```python
from build123d import *

# Parameters (mm, degrees)
F3_DEPTH       = 12
F8_R           = 1
F9_DEPTH       = 8
F10_R          = 4.5
F11_DEPTH      = 2
F12_R          = 1
F13_REACH      = 37.3532145158
F12_R_2        = 4.5
F14_DEPTH      = 6
F16_END_RADIUS = 1
F15_R          = 1
F16_REACH      = 37.3532145367
F15_R_2        = 4.5
F17_DEPTH      = 6
F19_END_RADIUS = 1
F18_R          = 1
F19_REACH      = 37.3532145367
F18_R_2        = 4.5
F20_DEPTH      = 6
F22_DEPTH      = 25
F23_R          = 17.5
F23_R_2        = 1.5
F23_R_3        = 6.5
F23_R_4        = 4.5
F24_DEPTH      = 15
F25_DEPTH      = 10


with BuildPart() as f3:
    # F2 (on Top) → F3 (new body)
    with BuildSketch(Plane.XY):
        Polygon((25, -14.4337567297), (0, 28.8675134595), (-25, -14.4337567297), align=None)
    extrude(amount=-F3_DEPTH)

    # F3_face (on face) → F6 section 0
    with BuildSketch(Plane.XY, mode=Mode.PRIVATE) as f6_s0:
        Polygon((-25, -14.4337567297), (25, -14.4337567297), (0, 28.8675134595), align=None)
    loft([f6_s0.sketch, Vertex(0, 0, 10)])

    # F8 (on face) → F9 (cut)
    with BuildSketch(Plane(origin=(0, 0, -12), x_dir=(1, 0, 0), z_dir=(0, 0, -1))):
        Circle(F8_R)
    extrude(amount=-F9_DEPTH, mode=Mode.SUBTRACT)

    # F10 (on face) → F11 (cut)
    with BuildSketch(Plane(origin=(0, 0, -12), x_dir=(1, 0, 0), z_dir=(0, 0, -1))):
        Circle(F10_R)
    extrude(amount=-F11_DEPTH, mode=Mode.SUBTRACT)

    f13_end = f3.faces().sort_by_distance((-1, 0, -7))[0]
    # F12 (on face) → F13 (cut, up to a face of the model that its end follows)
    with BuildSketch(Plane(origin=(0, -4.6812183988, 6.7567567568), x_dir=(1, 0, 0), z_dir=(0, -0.5694947975, 0.8219949365))):
        with Locations((0, -4.3050520255)):
            Circle(F12_R)
    f13_long = extrude(amount=-F13_REACH, mode=Mode.PRIVATE)
    add(split(f13_long, bisect_by=f13_end, keep=Keep.BOTTOM, mode=Mode.PRIVATE), mode=Mode.SUBTRACT)

    # F12 (on face) → F14 (cut)
    with BuildSketch(Plane(origin=(0, -4.6812183988, 6.7567567568), x_dir=(1, 0, 0), z_dir=(0, -0.5694947975, 0.8219949365))):
        with Locations((0, -4.3050520255)):
            Circle(F12_R_2)
        with Locations((0, -4.3050520255)):
            Circle(F12_R, mode=Mode.SUBTRACT)
    extrude(amount=-F14_DEPTH, mode=Mode.SUBTRACT)

    f16_end = (Plane(origin=(0, 0, -7), x_dir=(-1, 0, 0), z_dir=(0, 0, -1)) * Cylinder(F16_END_RADIUS, 214.1194850146, mode=Mode.PRIVATE)).faces().sort_by_distance((-1, 0, -7))[0]
    # F15 (on face) → F16 (cut, up to the whole of a round face its end follows)
    with BuildSketch(Plane(origin=(-4.0540540541, 2.3406091994, 6.7567567568), x_dir=(0.8699176724, 0.1614366008, 0.4660273245), z_dir=(-0.4931969619, 0.2847473987, 0.8219949365))):
        with Locations((-3.5228976388, 2.474401982)):
            Circle(F15_R)
    f16_long = extrude(amount=-F16_REACH, mode=Mode.PRIVATE)
    add(split(f16_long, bisect_by=f16_end, keep=Keep.ALL, mode=Mode.PRIVATE).solids().sort_by_distance((-7.1186849681, 4.1099746826, 4.3050520255))[0], mode=Mode.SUBTRACT)

    # F15 (on face) → F17 (cut)
    with BuildSketch(Plane(origin=(-4.0540540541, 2.3406091994, 6.7567567568), x_dir=(0.8699176724, 0.1614366008, 0.4660273245), z_dir=(-0.4931969619, 0.2847473987, 0.8219949365))):
        with Locations((-3.5228976388, 2.474401982)):
            Circle(F15_R_2)
        with Locations((-3.5228976388, 2.474401982)):
            Circle(F15_R, mode=Mode.SUBTRACT)
    extrude(amount=-F17_DEPTH, mode=Mode.SUBTRACT)

    f19_end = (Plane(origin=(0, 0, -7), x_dir=(-1, 0, 0), z_dir=(0, 0, -1)) * Cylinder(F19_END_RADIUS, 214.1194850146, mode=Mode.PRIVATE)).faces().sort_by_distance((-1, 0, -9.9336675042))[0]
    # F18 (on face) → F19 (cut, up to the whole of a round face its end follows)
    with BuildSketch(Plane(origin=(4.0540540541, 2.3406091994, 6.7567567568), x_dir=(0.8699176724, -0.1614366008, -0.4660273245), z_dir=(0.4931969619, 0.2847473987, 0.8219949365))):
        with Locations((3.5228976388, 2.474401982)):
            Circle(F18_R)
    f19_long = extrude(amount=-F19_REACH, mode=Mode.PRIVATE)
    add(split(f19_long, bisect_by=f19_end, keep=Keep.ALL, mode=Mode.PRIVATE).solids().sort_by_distance((7.1186849681, 4.1099746826, 4.3050520255))[0], mode=Mode.SUBTRACT)

    # F18 (on face) → F20 (cut)
    with BuildSketch(Plane(origin=(4.0540540541, 2.3406091994, 6.7567567568), x_dir=(0.8699176724, -0.1614366008, -0.4660273245), z_dir=(0.4931969619, 0.2847473987, 0.8219949365))):
        with Locations((3.5228976388, 2.474401982)):
            Circle(F18_R_2)
        with Locations((3.5228976388, 2.474401982)):
            Circle(F18_R, mode=Mode.SUBTRACT)
    extrude(amount=-F20_DEPTH, mode=Mode.SUBTRACT)

    # F21 (on face) → F22 (cut)
    with BuildSketch(Plane(origin=(0, 0, -12), x_dir=(1, 0, 0), z_dir=(0, 0, -1))):
        with BuildLine():
            Line((3.2541491538, -23.2311617897), (7.5523574637, -15.7864466154))
            ThreePointArc((7.5523574637, -15.7864466154), (0, -17.5), (-7.5523574637, -15.7864466154))
            Line((-7.5523574637, -15.7864466154), (-3.2541491538, -23.2311617897))
            ThreePointArc((-3.2541491538, -23.2311617897), (0, -23.4579701768), (3.2541491538, -23.2311617897))
        make_face()
        with BuildLine():
            ThreePointArc((-9.8952850725, 14.4337567297), (0, 17.5), (9.8952850725, 14.4337567297))
            Line((9.8952850725, 14.4337567297), (18.4917016925, 14.4337567297))
            ThreePointArc((18.4917016925, 14.4337567297), (0, 23.4579701768), (-18.4917016925, 14.4337567297))
            Line((-18.4917016925, 14.4337567297), (-9.8952850725, 14.4337567297))
        make_face()
        with BuildLine():
            ThreePointArc((-17.4476425363, 1.3526898856), (-15.1554445662, 8.75), (-9.8952850725, 14.4337567297))
            Line((-9.8952850725, 14.4337567297), (-18.4917016925, 14.4337567297))
            ThreePointArc((-18.4917016925, 14.4337567297), (-20.3151980943, 11.7289850884), (-21.7458508462, 8.79740506))
            Line((-21.7458508462, 8.79740506), (-17.4476425363, 1.3526898856))
        make_face()
        with BuildLine():
            ThreePointArc((9.8952850725, 14.4337567297), (15.1554445662, 8.75), (17.4476425363, 1.3526898856))
            Line((17.4476425363, 1.3526898856), (21.7458508462, 8.79740506))
            ThreePointArc((21.7458508462, 8.79740506), (20.3151980943, 11.7289850884), (18.4917016925, 14.4337567297))
            Line((18.4917016925, 14.4337567297), (9.8952850725, 14.4337567297))
        make_face()
        with BuildLine():
            Line((0, -28.8675134595), (3.2541491538, -23.2311617897))
            ThreePointArc((3.2541491538, -23.2311617897), (0, -23.4579701768), (-3.2541491538, -23.2311617897))
            Line((-3.2541491538, -23.2311617897), (0, -28.8675134595))
        make_face()
        with BuildLine():
            ThreePointArc((-21.7458508462, 8.79740506), (-20.3151980943, 11.7289850884), (-18.4917016925, 14.4337567297))
            Line((-18.4917016925, 14.4337567297), (-25, 14.4337567297))
            Line((-25, 14.4337567297), (-21.7458508462, 8.79740506))
        make_face()
        with BuildLine():
            ThreePointArc((18.4917016925, 14.4337567297), (20.3151980943, 11.7289850884), (21.7458508462, 8.79740506))
            Line((21.7458508462, 8.79740506), (25, 14.4337567297))
            Line((25, 14.4337567297), (18.4917016925, 14.4337567297))
        make_face()
    extrude(amount=-F22_DEPTH, mode=Mode.SUBTRACT)

    # F23 (on face) → F24 (join)
    with BuildSketch(Plane(origin=(0, 0, -12), x_dir=(1, 0, 0), z_dir=(0, 0, -1))):
        Circle(F23_R)
        with Locations((-10.8253175473, -6.25)):
            Circle(F23_R_2, mode=Mode.SUBTRACT)
        Circle(F23_R_3, mode=Mode.SUBTRACT)
        with Locations((10.8253175473, 6.25)):
            Circle(F23_R_2, mode=Mode.SUBTRACT)
        Circle(F23_R_3)
        Circle(F23_R_4, mode=Mode.SUBTRACT)
    extrude(amount=F24_DEPTH)

    # F25 (add): a face of the model
    f25_faces = [f3.faces().sort_by_distance(p)[0] for p in [
        (-4.3727207794, 0, -10),
    ]]
    extrude(f25_faces, amount=F25_DEPTH)


solid = f3.part
```
Check sheet for the modelled part. Datum: model origin and axes. Units: mm. A direction names the side the tool comes from. Round coordinates to 2 decimals unless told otherwise and drop trailing zeros. Loops run counter-clockwise (first coordinate to the right, second up) from the corner with the lowest first, then second, coordinate; pieces in that order, holes last. Notation, with made-up numbers: (17.5, 46.5) - (60.5, 46.5) arc R25 cw to (60.5, 79.5) - close; hole circle Ø8 at (-26, 36). An arc over 180 degrees is marked (long way). Answer as a JSON object with one key per item and string values. Group by question number.
Q1. Sectioned sample at D-D, the plane x = 3. Count the separate pieces of the cut face and the enclosed holes in it, plus the area to 3 significant figures.
Q2. Mould release check, pull along Z, two halves, no side actions. Record for faces 1 (the face through (14, 8, -12)), 2 (the face through (2.98, 1.37, -4.52)), 3 (the face through (0.94, -5.57, -1.16)), 4 (the face through (12.569, 7.097, -5.916)): released by +Z, released by -Z, zero draft, split by the parting line, or undercut.
Q3. Sectioned sample at A-A, the plane z = -11. Enter the section's corners in (x, y), plus the area to 3 significant figures.
Q4. Set-up check for faces 5 (the face through (0, -14.434, -6)), 6 (the face through (1, 1, -20)), 7 (the face through (-3.34, 1.67, 0.12)), 8 (the face through (-14, 8, -12)): record each of +Z, -Z, +X, -X, +Y, -Y from which the full face is reachable in a straight line by a thin tool's end or side.
Q5. Sectioned sample at C-C, the plane x = -14. Enter the section's corners in (y, z), plus the area to 3 significant figures.
Q6. Gauge pin test, flat ends, axial feed: P1, Ø1.5, axis at y = -3, z = 6, coming from the +X side; P2, Ø1.6, axis at x = -0.5, y = 0, coming from the -Z side; P3, Ø1, axis at x = -8.5, z = -23, coming from the +Y side. Record the tip position at first contact, or that the pin passes through.
Q7. Sectioned sample at B-B, the plane y = 13.5. Enter the section's corners in (x, z), plus the area to 3 significant figures.
Q8. Scan lines: line 1 along Y through (x, z) = (0, -14); line 2 along Z through (x, y) = (-3, 1.5); line 3 along Y through (x, z) = (0, -22). Record each from-to range of solid material in increasing order. Write a range as [from, to].
Solution:
{
 "1": {"separate pieces": "1", "enclosed holes": "2", "area": "924 mm²"},
 "2": {"face 1": "released by +Z", "face 2": "undercut", "face 3": "undercut", "face 4": "zero draft"},
 "3": {"outline": "(-17.45, -1.35) arc R17.5 ccw to (-9.9, -14.43) - (9.9, -14.43) arc R17.5 ccw to (17.45, -1.35) - (7.55, 15.79) arc R17.5 ccw to (-7.55, 15.79) - close; hole circle Ø2 at (0, 0)", "area": "835 mm²"},
 "4": {"face 5": "+Z, +X, -X, -Y", "face 6": "-Z", "face 7": "none", "face 8": "+Z, -X, +Y"},
 "5": {"outline": "(-10.5, -27) - (10.5, -27) - (10.5, -12) - (4.62, -12) - (4.62, 0) - (-8.08, 4.4) - (-10.5, 2.73) - close", "area": "533 mm²"},
 "6": {"P1": "stops at x = 9.72", "P2": "stops at z = -20", "P3": "stops at y = 15.56"},
 "7": {"outline": "(-11.14, -27) - (11.14, -27) - (11.14, -12) - (8.87, -12) - (8.87, 0) - (0, 5.32) - (-8.87, 0) - (-8.87, -12) - (-11.14, -12) - close", "area": "594 mm²"},
 "8": {"line 1": "y = [-17.5, -1], [1, 17.5]", "line 2": "z = [-20, -4.45], [-1.01, 0.38], [5.17, 7.68]", "line 3": "y = [-17.5, -4.5], [4.5, 17.5]"}
}
